For this review, use the dimensioned drawing (mm, ordinates from the lowest corner) and the shaded views. A direction names the side the tool comes from. Round coordinates to 2 decimals unless told otherwise and drop trailing zeros. Order: outer loops, then holes, each group sorted by start corner. A loop starts at its lowest first (then second) coordinate and runs counter-clockwise, first axis right, second up. Notation, with made-up numbers: (84, 37) -> (135, 37) arc R23 ccw to (135, 51) -> close; hole circle Ø8 at (71.5, -34). An arc over 180 degrees is marked (long way). Use a Markdown table: item, result. Add a question column.
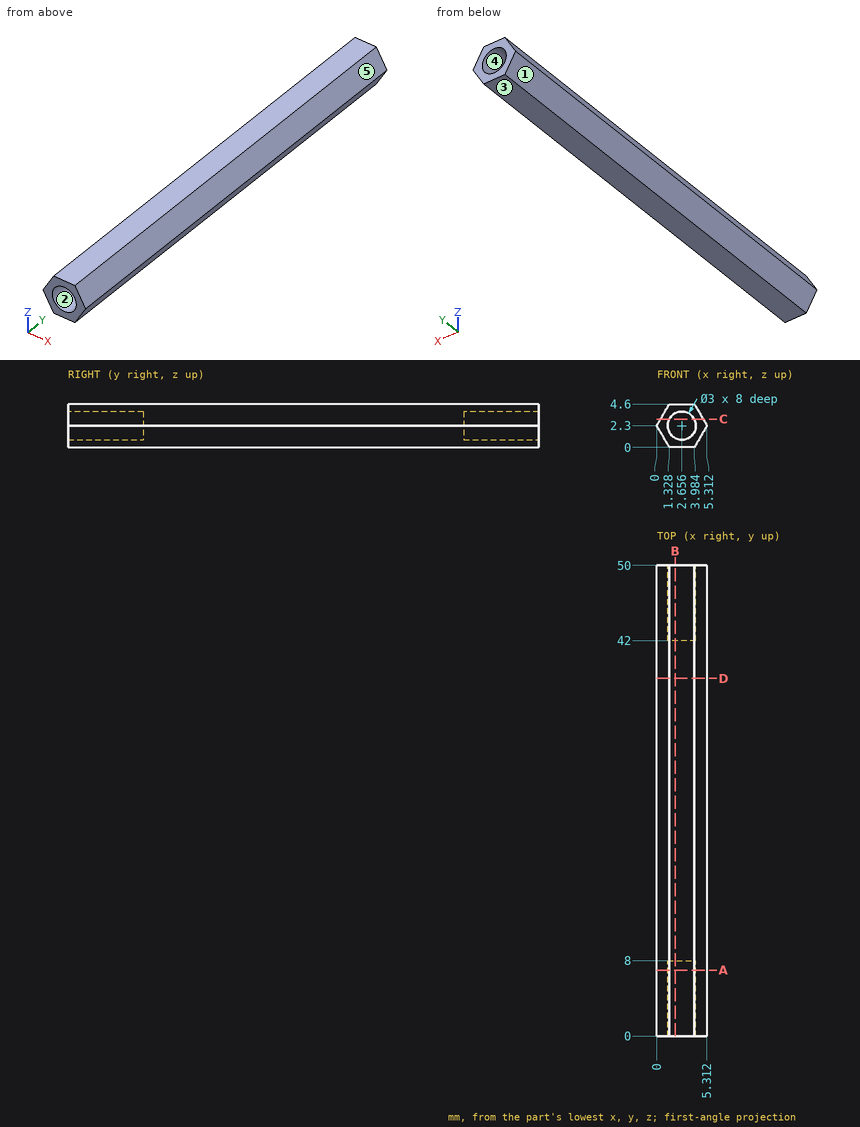
Q1. Add section D-D (y = 38). Write out the cut boundary in (x, z).
Q2. Wall thickness on line 1 (X direction, y = 46.25, z = 2.3) (1 decimal); line 2 (X direction, y = 45.5, z = 3.65) (1 decimal); line 3 (Z direction, x = 1.4, y = 7.5): over which ranges is each line inside the solid? List them lowest first. Write a range as [from, to].
Q3. Insertion check: pin 1 (1.8 mm diameter, centred on x = 2.66, z = 2.3, fed in from -Y); pin 2 (0.9 mm diameter, centred on x = 3, z = 2, fed in from +Y). Each pin has a flat end and moves straight along its axis. Give the tip position at first contact, or say it passes through.
Q4. Add section A-A (y = 7). Write out the cut boundary in (x, z).
Q5. Machinability: for the marked faces 1 and 2, which of the approach directions +Z, -Z, +X, -X, +Y, -Y give a long, thin tool a straight path to every point of the face, cutting with its end or side? Answer none if there is none.
Q6. Add section B-B (x = 1.95). Write out the cut boundary in (y, z).
Q7. Add section C-C (z = 3). Write out the cut boundary in (x, y), then the cut area to 3 significant figures.
Q8. Mouldability with a two-part tool opening along X and no side actions: class the marked faces 3, 4 and 5 as pulls with the +X half, pulls with the -X half, needs draft (parallel to the pull), parting line crosses it, or undercut.
Report:
| question | item | result |
|---|---|---|
| 1 | outline | (0, 2.3) -> (1.33, 0) -> (3.98, 0) -> (5.31, 2.3) -> (3.98, 4.6) -> (1.33, 4.6) -> close |
| 2 | line 1 | x = [0, 1.2], [4.2, 5.3] |
| 2 | line 2 | x = [0.8, 2], [3.3, 4.5] |
| 2 | line 3 | z = [0, 1.48], [3.12, 4.6] |
| 3 | pin 1 | stops at y = 8 |
| 3 | pin 2 | stops at y = 42 |
| 4 | outline | (0, 2.3) -> (1.33, 0) -> (3.98, 0) -> (5.31, 2.3) -> (3.98, 4.6) -> (1.33, 4.6) -> close; hole circle Ø3 at (2.66, 2.3) |
| 5 | face 1 | -Z, -X, +Y, -Y |
| 5 | face 2 | -Y |
| 6 | outline | (0, 0) -> (50, 0) -> (50, 0.98) -> (42, 0.98) -> (42, 3.62) -> (50, 3.62) -> (50, 4.6) -> (0, 4.6) -> (0, 3.62) -> (8, 3.62) -> (8, 0.98) -> (0, 0.98) -> close |
| 7 | outline | (0.4, 0) -> (1.33, 0) -> (1.33, 8) -> (3.98, 8) -> (3.98, 0) -> (4.91, 0) -> (4.91, 50) -> (3.98, 50) -> (3.98, 42) -> (1.33, 42) -> (1.33, 50) -> (0.4, 50) -> close |
| 7 | area | 183 mm² |
| 8 | face 3 | needs draft |
| 8 | face 4 | undercut |
| 8 | face 5 | pulls with the +X half |
